Study the drawing (mm; zero at the part's minimum x, y, z) and answer. A direction names the side the tool comes from. Coordinates: 2 decimals unless noted, no trailing zeros. Loops run counter-clockwise (first coordinate to the right, second up) from the corner with the lowest first, then second, coordinate; pieces in that order, holes last. Notation, with made-up numbers: (48, 86.5) -> (82, 86.5) arc R21 cw to (82, 114.5) -> close; hole circle Ø11 at (65, 75.5). An arc over 180 degrees is marked (long way). Answer as CSV lines item,"result".
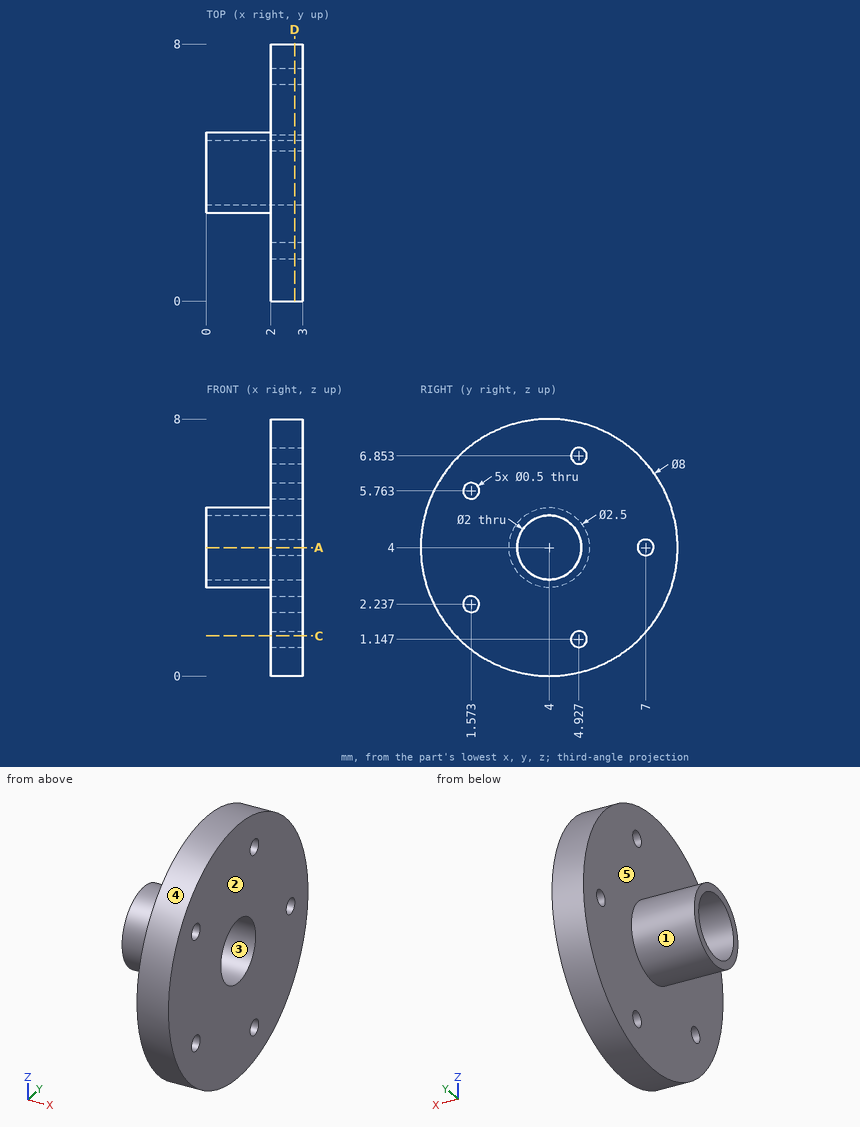
Q1. For a pull along Y with two mould halves and no side action, classify the marked faces 1, 2 and 3 as pulls with the +Y half, pulls with the -Y half, needs draft (parallel to the pull), parting line crosses it, or undercut.
Results:
face 1,"parting line crosses it"
face 2,"needs draft"
face 3,"undercut"
Q2. A cutting plane is placed at D-D, the plane x = 2.75. Give the number of separate pieces and of enclosed holes in the cut face.
Results:
separate pieces,"1"
enclosed holes,"6"
Q3. For the marked faces 4 and 5, determine the directions among +Z, -Z, +X, -X, +Y, -Y from which every point of the face is accessible in a straight line to the end or side of a thin tool.
Results:
face 4,"+X, -X"
face 5,"-X"
Q4. A cutting plane is placed at C-C, the plane z = 1.25. Write down the section's boundary in (x, y) (1 decimal).
Results:
outline,"(2, 1.1) -> (3, 1.1) -> (3, 4.7) -> (2, 4.7) -> close; (2, 5.2) -> (3, 5.2) -> (3, 6.9) -> (2, 6.9) -> close"
Q5. Find the intervals of material crossed by probe 1 along Y at (x, z) = (1.4, 4); probe 2 along X at (y, z) = (6.75, 2), in increasing order. Write a range as [from, to].
Results:
probe 1,"y = [2.75, 3], [5, 5.25]"
probe 2,"x = [2, 3]"
Q6. A cutting plane is placed at A-A, the plane z = 4. Write down the section's boundary in (x, y).
Results:
outline,"(0, 2.75) -> (2, 2.75) -> (2, 0) -> (3, 0) -> (3, 3) -> (0, 3) -> close; (0, 5) -> (3, 5) -> (3, 6.75) -> (2, 6.75) -> (2, 5.25) -> (0, 5.25) -> close; (2, 7.25) -> (3, 7.25) -> (3, 8) -> (2, 8) -> close"
Q7. Given pin 1 Ø1 at (x, z) = (2, 1) entering from +Y; pin 2 Ø1.2 at (y, z) = (4, 4) entering from -X; pin 3 Ø1.5 at (x, y) = (1.5, 2) entering from -Z, each flat-ended and moving along its own axis, determine where each tip first touches the part or whether it passes through.
Results:
pin 1,"stops at y = 7.12"
pin 2,"passes through"
pin 3,"stops at z = 0.27"
